Build history of the part. All positions in model axes, mm. A direction names the side the tool comes from. Give positions to 0.01 mm unless a question says otherwise; leave off trailing zeros. Order: outer loops, then holes, each group sorted by start corner. A loop starts at its lowest first (then second) coordinate and runs counter-clockwise, first axis right, second up. Notation, with made-up numbers: (84.5, -40) -> (123.5, -40) arc R22 ccw to (123.5, -6) -> close; hole circle Ø6 at (86.25, 83.25). An arc over 180 degrees is marked (long way). One line per item, written item: value. Start each with the question number.
(1) Which spindle directions (+Z, -Z, +X, -X, +Y, -Y) get a long thin tool onto all of the face, cutting with end or side? Do faces 5 (the flat face through (14, 2, -10)), 6 (the flat face through (48, 10, -8)), 7 (the cylindrical face through (-69.874, 4.715, -14.846)). Say none if no direction does.
(2) Saw through at A-A on y = 7.25. Give the cut face in (x, z).
(3) Two-plate mould, pull along Z, no slides. Class faces 1 (the flat face through (-84, 0, -30.389)), 2 (the flat face through (48, 10, -2)), 3 (the cylindrical face through (32.11, -0.07, -6.34)), 4 (the flat face through (55, 1, -5)): +Z half, -Z half, draft (parallel to the pull), parting line (faces both ways), or undercut.
(4) Pin check, flat tips, straight feed: pin 1 (10.5 mm diameter, centred on x = 0.5, y = 9.5, fed in from -Z); pin 2 (1 mm diameter, centred on y = 13.5, z = -0.5, fed in from +X); pin 3 (3 mm diameter, centred on x = -0.5, z = 1, fed in from -Y); pin 4 (1 mm diameter, centred on x = 51, z = -1, fed in from +Y). Stop position of each tip, or through.
(5) Saw through at B-B on x = 30. Give the cut face in (y, z), plus the area to 3 significant figures.
(6) Saw through at C-C on x = -29. Give the cut face in (y, z), plus the area to 3 significant figures.
(7) Probe line 1 (X direction, y = 1, z = -5); line 2 (X direction, y = -2, z = -1); line 3 (Z direction, x = 13, y = 0.75). List the from-to ranges inside material, lowest first.
```python
from build123d import *

# Parameters (mm, degrees)
BOSS_EXTRUDE2_DEPTH = 5
SKETCH3_W           = 14
SKETCH3_H           = 5
SKETCH3_W_2         = 10
SKETCH3_H_2         = 7
BOSS_EXTRUDE3_DEPTH = 2
SKETCH4_R           = 1
CUT_EXTRUDE1_DEPTH  = 96.580030811
FILLET1_R           = 1
FILLET2_R           = 1
SKETCH5_R           = 2.5
CUT_EXTRUDE2_DEPTH  = 97.594732206
BOSS_EXTRUDE4_DEPTH = 5


with BuildPart() as part:
    # Sketch1 → Boss-Extrude2 (new, symmetric)
    with BuildSketch(Plane(origin=(0, 0, 0), x_dir=(1, 0, 0), z_dir=(0, 1, 0))):
        with BuildLine():
            Line((-49, 0), (49, 0))
            Line((49, 0), (55, 0))
            Line((55, 0), (55, 10))
            Line((55, 10), (49, 10))
            Line((49, 10), (-48.597064799, 10))
            ThreePointArc((-48.597064799, 10), (-51.770174838, 10.516784686), (-54.615321941, 12.013725463))
            Line((-54.615321941, 12.013725463), (-78.198331144, 29.785292532))
            ThreePointArc((-78.198331144, 29.785292532), (-79.051875275, 30.234374765), (-80.003808287, 30.389410171))
            Line((-80.003808287, 30.389410171), (-88.011381516, 30.389410171))
            ThreePointArc((-88.011381516, 30.389410171), (-88.959703047, 29.706721175), (-88.61320723, 28.590782717))
            Line((-88.61320723, 28.590782717), (-52.009128571, 1.006862732))
            ThreePointArc((-52.009128571, 1.006862732), (-50.586555019, 0.258392343), (-49, 0))
        make_face()
    extrude(amount=BOSS_EXTRUDE2_DEPTH, both=True)

    # Sketch3 → Boss-Extrude3 (add)
    with BuildSketch(Plane.XY):
        with Locations((48, 7.5)):
            Rectangle(SKETCH3_W, SKETCH3_H)
        with Locations((48, 13.5)):
            Rectangle(SKETCH3_W_2, SKETCH3_H_2)
    boss_extrude3 = extrude(amount=-BOSS_EXTRUDE3_DEPTH)

    # Sketch4 → Cut-Extrude1 (cut, through all)
    with BuildSketch(Plane.XY):
        with BuildLine():
            ThreePointArc((41, 9), (41.292893219, 9.707106781), (42, 10))
            Line((42, 10), (41, 10))
            Line((41, 10), (41, 9))
        make_face()
        with BuildLine():
            Line((43, 17), (43, 10))
            Line((43, 10), (48.581791004, 16.103269862))
            ThreePointArc((48.581791004, 16.103269862), (49.441268366, 16.764748844), (50.5, 17))
            Line((50.5, 17), (43, 17))
        make_face()
        with BuildLine():
            Line((52.267766953, 12.732233047), (49.768982827, 10))
            Line((49.768982827, 10), (53, 10))
            Line((53, 10), (53, 14.5))
            ThreePointArc((53, 14.5), (52.809698831, 13.543291419), (52.267766953, 12.732233047))
        make_face()
        with BuildLine():
            Line((53, 17), (50.5, 17))
            ThreePointArc((50.5, 17), (52.267766953, 16.267766953), (53, 14.5))
            Line((53, 14.5), (53, 17))
        make_face()
        with BuildLine():
            Line((55, 10), (54, 10))
            ThreePointArc((54, 10), (54.707106781, 9.707106781), (55, 9))
            Line((55, 9), (55, 10))
        make_face()
        with Locations((50.5, 14.5)):
            Circle(SKETCH4_R)
    cut_extrude1 = extrude(amount=-CUT_EXTRUDE1_DEPTH, mode=Mode.SUBTRACT)

    # Mirror1: Boss-Extrude3, Cut-Extrude1 across plane
    add(boss_extrude3.mirror(Plane.XY.offset(-5)))
    add(cut_extrude1.mirror(Plane.XY.offset(-5)), mode=Mode.SUBTRACT)

    # Fillet1
    fillet1_edges = [part.edges().sort_by_distance(p)[0] for p in [
        (3, -5, 0),
        (-50.586555019, -5, -0.258392343),
        (-70.3111679, -5, -14.798822724),
        (-88.959703047, -5, -29.706721175),
        (-84.007594901, -5, -30.389410171),
        (-79.051875275, -5, -30.234374765),
        (-66.406826543, -5, -20.899508998),
        (-51.770174838, -5, -10.516784686),
        (3.2014676, -5, -10),
    ]]
    fillet(fillet1_edges, radius=FILLET1_R)

    # Fillet2
    fillet2_edges = [part.edges().sort_by_distance(p)[0] for p in [
        (-3.7985324, 5, -10),
        (-51.770174838, 5, -10.516784686),
        (-66.406826543, 5, -20.899508998),
        (-79.051875275, 5, -30.234374765),
        (-84.007594901, 5, -30.389410171),
        (-88.959703047, 5, -29.706721175),
        (-70.3111679, 5, -14.798822724),
        (-50.586555019, 5, -0.258392343),
        (-4, 5, 0),
    ]]
    fillet(fillet2_edges, radius=FILLET2_R)

    # Sketch5 → Cut-Extrude2 (cut, through all)
    with BuildSketch(Plane.XZ.offset(5)):
        with Locations(Location((-35, -5, 0), (0, 0, 270))):
            Circle(SKETCH5_R)
        with Locations(Location((30, -5, 0), (0, 0, 270))):
            Circle(SKETCH5_R)
    extrude(amount=-CUT_EXTRUDE2_DEPTH, mode=Mode.SUBTRACT)

    # Sketch8 → Boss-Extrude4 (add, symmetric)
    with BuildSketch(Plane(origin=(0, 0, 0), x_dir=(0, 0, -1), z_dir=(1, 0, 0))):
        with BuildLine():
            Line((0, 2.75), (0, -2.75))
            Line((0, -2.75), (-2.75, -2.75))
            ThreePointArc((-2.75, -2.75), (-4.694543648, -1.944543648), (-5.5, 0))
            Line((-5.5, 0), (-5, 0))
            ThreePointArc((-5, 0), (-4.340990258, -1.590990258), (-2.75, -2.25))
            ThreePointArc((-2.75, -2.25), (-0.5, 0), (-2.75, 2.25))
            Line((-2.75, 2.25), (-2.75, 2.75))
            Line((-2.75, 2.75), (0, 2.75))
        make_face()
    extrude(amount=BOSS_EXTRUDE4_DEPTH, both=True)


solid = part.part
```
Results below:
1. face 5: -Z, +X, +Y, -Y
1. face 6: +X, -X, +Y
1. face 7: +Z, -X, +Y
2. outline: (41, -10) -> (55, -10) -> (55, -8) -> (41, -8) -> close; (41, -2) -> (55, -2) -> (55, 0) -> (41, 0) -> close
3. face 1: -Z half
3. face 2: undercut
3. face 3: undercut
3. face 4: draft
4. pin 1: stops at z = -9.97
4. pin 2: stops at x = 52.95
4. pin 3: stops at y = -4.87
4. pin 4: stops at y = 17
5. outline: (-5, -9) arc R1 ccw to (-4, -10) -> (4, -10) arc R1 ccw to (5, -9) -> (5, -7.5) -> (-5, -7.5) -> close; (-5, -2.5) -> (5, -2.5) -> (5, -1) arc R1 ccw to (4, 0) -> (-4, 0) arc R1 ccw to (-5, -1) -> close
5. area: 49.1 mm²
6. outline: (-5, -9) arc R1 ccw to (-4, -10) -> (4, -10) arc R1 ccw to (5, -9) -> (5, -1) arc R1 ccw to (4, 0) -> (-4, 0) arc R1 ccw to (-5, -1) -> close
6. area: 99.1 mm²
7. line 1: x = -57.31 to -37.5, -32.5 to 27.5, 32.5 to 55
7. line 2: x = -52 to 55
7. line 3: z = -10 to 0
